The listing builds one solid part. Answer for the finished solid, in the listing's coordinates (mm). A direction names the side the tool comes from. Round coordinates to 2 decimals unless told otherwise and drop trailing zeros. Write each loop counter-clockwise with the first axis right and the second up, starting at its lowest first coordinate (ties: lowest second). Pieces come first, ordered by that corner, then holes. Notation, with made-up numbers: (56.25, 14) - (85.25, 14) arc R30 ccw to (85.25, 53) - close; hole circle Ø8 at (-38.5, -19). An arc over 180 degrees is marked (long way). Answer in a Markdown table with one row per item.
from build123d import *

# Parameters (mm, degrees)
F0_R     = 76.2
F0_R_2   = 8.89
F1_DEPTH = 19.05
F2_R     = 39.6875
F2_R_2   = 33.02
F3_DEPTH = 19.05
F4_R     = 33.02
F5_DEPTH = 25.4


with BuildPart() as f1:
    # F0 (on Front) → F1 (new body)
    with BuildSketch(Plane.XZ):
        Circle(F0_R)
        with Locations((-46.743721, -26.9875)):
            Circle(F0_R_2, mode=Mode.SUBTRACT)
        with Locations((0, -53.975)):
            Circle(F0_R_2, mode=Mode.SUBTRACT)
        with Locations((46.743721, -26.9875)):
            Circle(F0_R_2, mode=Mode.SUBTRACT)
        with Locations((-46.743721, 26.9875)):
            Circle(F0_R_2, mode=Mode.SUBTRACT)
        with Locations((46.743721, 26.9875)):
            Circle(F0_R_2, mode=Mode.SUBTRACT)
        with Locations((0, 53.975)):
            Circle(F0_R_2, mode=Mode.SUBTRACT)
    extrude(amount=F1_DEPTH)

    # F2 (on face) → F3 (join)
    with BuildSketch(Plane.XZ.offset(19.05)):
        Circle(F2_R)
        Circle(F2_R_2, mode=Mode.SUBTRACT)
    extrude(amount=F3_DEPTH)

    # F4 (on face) → F5 (cut)
    with BuildSketch(Plane.XZ.offset(19.05)):
        Circle(F4_R)
    extrude(amount=-F5_DEPTH, mode=Mode.SUBTRACT)


solid = f1.part
(1) Find the intervals of material crossed by line 1 (Z direction, x = 0, y = -6.5) (3 decimals); line 2 (X direction, y = -7.5, z = -1.5); line 3 (Z direction, x = 0, y = -33), in increasing order.
Checked values:
| item | result |
|---|---|
| line 1 | z = -76.2 to -62.865, -45.085 to -33.02, 33.02 to 45.085, 62.865 to 76.2 |
| line 2 | x = -76.19 to -32.99, 32.99 to 76.19 |
| line 3 | z = -39.69 to -33.02, 33.02 to 39.69 |
(2) Section B-B (x = 0) is taken. State how many separate pieces and enclosed holes the cut face has, and give its area (3 significant figures).
Checked values:
| item | result |
|---|---|
| separate pieces | 4 |
| enclosed holes | 0 |
| area | 1,220 mm2 |
(3) For faces 4 (the cylindrical face through (-55.625, -9.392, 27.378)), 5 (the flat face through (33, -19.05, -33)), determine the directions among +Z, -Z, +X, -X, +Y, -Y from which every point of the face is accessible in a straight line to the end or side of a thin tool.
Checked values:
| item | result |
|---|---|
| face 4 | +Y, -Y |
| face 5 | -Y |
(4) For a pull along X with two mould halves and no side action, classify faces 1 (the cylindrical face through (-1.927, -9.392, -62.654)), 2 (the flat face through (-15, -38.1, 30)), 3 (the cylindrical face through (-60.47, -9.392, -46.367)) as pulls with the +X half, pulls with the -X half, needs draft (parallel to the pull), parting line crosses it, or undercut.
Checked values:
| item | result |
|---|---|
| face 1 | undercut |
| face 2 | needs draft |
| face 3 | parting line crosses it |
(5) Section C-C (y = -3) is taken. Give the vertices of the cut face in (x, z) (1 decimal), and give its area (3 significant figures).
Checked values:
| item | result |
|---|---|
| outline | circle Ø152.4 at (0, 0); hole circle Ø17.8 at (-46.7, -27); hole circle Ø17.8 at (-46.7, 27); hole circle Ø66 at (0, 0); hole circle Ø17.8 at (0, -54); hole circle Ø17.8 at (0, 54); hole circle Ø17.8 at (46.7, -27); hole circle Ø17.8 at (46.7, 27) |
| area | 13,300 mm2 |
(6) Section A-A (z = 0) is taken. Give the vertices of the cut face in (x, y), and give its area (3 significant figures).
Checked values:
| item | result |
|---|---|
| outline | (-76.2, -19.05) - (-39.69, -19.05) - (-39.69, -38.1) - (-33.02, -38.1) - (-33.02, 0) - (-76.2, 0) - close; (33.02, -38.1) - (39.69, -38.1) - (39.69, -19.05) - (76.2, -19.05) - (76.2, 0) - (33.02, 0) - close |
| area | 1,900 mm2 |
(7) Section D-D (x = 22.5) is taken. Give the vertices of the cut face in (y, z), and give its area (3 significant figures).
Checked values:
| item | result |
|---|---|
| outline | (-38.1, -32.69) - (-19.05, -32.69) - (-19.05, -72.8) - (0, -72.8) - (0, -24.17) - (-38.1, -24.17) - close; (-38.1, 24.17) - (0, 24.17) - (0, 72.8) - (-19.05, 72.8) - (-19.05, 32.69) - (-38.1, 32.69) - close |
| area | 2,180 mm2 |
(8) Flat-ended cylindrical pins translate along their axes: pin 1 (3 mm diameter, centred on y = -26.5, z = -12, fed in from -X); pin 2 (1.5 mm diameter, centred on y = -22, z = -15, fed in from +X); pin 3 (5 mm diameter, centred on x = 31.5, y = -31, fed in from +Z); pin 4 (10.5 mm diameter, centred on x = -46.74, z = -26.99, fed in from +Y). Find the tip coordinate at first contact, or state that the pin passes through.
Checked values:
| item | result |
|---|---|
| pin 1 | stops at x = -38.27 |
| pin 2 | stops at x = 37.04 |
| pin 3 | stops at z = 27.09 |
| pin 4 | passes through |
